Design review of the part built by this model. Coordinates are the model's own, in mm. Round coordinates to 2 decimals unless told otherwise and drop trailing zeros. Loops run counter-clockwise (first coordinate to the right, second up) from the corner with the lowest first, then second, coordinate; pieces in that order, holes last. Notation, with made-up numbers: (-21, 75) - (35, 75) arc R19 ccw to (35, 80) - close; hole circle Ø10 at (-25.75, 63.25). An arc over 180 degrees is marked (long way). Return JSON: item names as keys, results as strings. Group by question number.
(1) Wall thickness on L1, parallel to Y at x = 48, z = 4.7; L2, parallel to Y at x = -96, z = 2.35; L3, parallel to X at y = 65.5, z = 1.4: over which ranges is each line inside the solid? List them lowest first. Write a range as [from, to].
(2) We need section C-C, the plane x = 0. Write out the cut boundary in (y, z), and give its area (3 significant figures).
(3) We need section A-A, the plane x = -96. Write out the cut boundary in (y, z).
(4) Clearance check with flat-ended pins moving along their axes: pin 1 (1.8 mm diameter, centred on x = 29.5, z = 4.5, fed in from -Y); pin 2 (1 mm diameter, centred on y = -33.5, z = 4.5, fed in from -X); pin 3 (1.8 mm diameter, centred on y = -31.5, z = 4, fed in from +X). State where each tip first meets the part, or that it passes through.
(5) We need section B-B, the plane z = 1.75. Write out the cut boundary in (x, y).
(6) We need section D-D, the plane y = 63. Write out the cut boundary in (x, z), and give its area (3 significant figures).
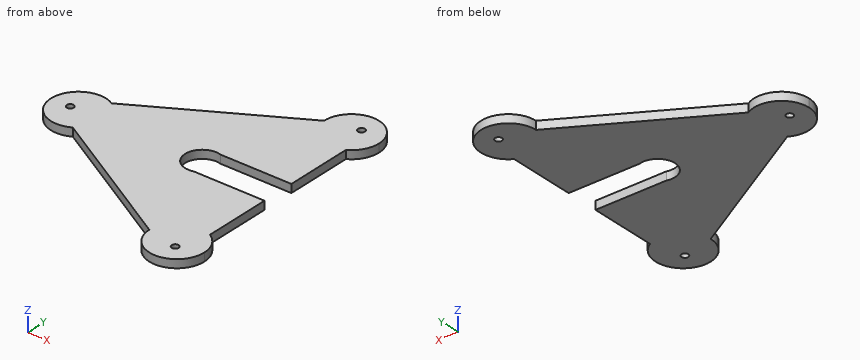
from build123d import *

# Parameters (mm, degrees)
F1_DEPTH        = 6
F2_R            = 12.5
F3_DEPTH        = 6
F4_R            = 2.5
F5_DEPTH        = 6
F5_COPIES_COUNT = 3
F6_W            = 60
F6_H            = 24
F7_DEPTH        = 6


# Not quite as in the source:
# - a pattern or mirror of a feature is missing from the dataset's text; its kind, count and spacing are read off the source's solid


with BuildPart() as f1:
    # F0 (on Top) → F1 (new body)
    with BuildSketch(Plane.XY):
        with BuildLine():
            ThreePointArc((-80, 17.3205080757), (-100, 17.3205080757), (-110, 0))
            Line((-110, 0), (-80, 17.3205080757))
        make_face()
        with BuildLine():
            Line((-80, 17.3205080757), (-110, 0))
            Line((-110, 0), (-80, -17.3205080757))
            ThreePointArc((-80, -17.3205080757), (-72.6794919243, -10), (-70, 0))
            ThreePointArc((-70, 0), (-72.6794919243, 10), (-80, 17.3205080757))
        make_face()
        with BuildLine():
            Line((-80, -17.3205080757), (-110, 0))
            ThreePointArc((-110, 0), (-100, -17.3205080757), (-80, -17.3205080757))
        make_face()
        with BuildLine():
            Line((25, 77.9422863406), (-80, 17.3205080757))
            ThreePointArc((-80, 17.3205080757), (-72.6794919243, 10), (-70, 0))
            ThreePointArc((-70, 0), (-72.6794919243, -10), (-80, -17.3205080757))
            Line((-80, -17.3205080757), (25, -77.9422863406))
            ThreePointArc((25, -77.9422863406), (35, -60.6217782649), (55, -60.6217782649))
            Line((55, -60.6217782649), (55, 60.6217782649))
            ThreePointArc((55, 60.6217782649), (35, 60.6217782649), (25, 77.9422863406))
        make_face()
        with BuildLine():
            ThreePointArc((55, 95.2627944163), (35, 95.2627944163), (25, 77.9422863406))
            Line((25, 77.9422863406), (55, 95.2627944163))
        make_face()
        with BuildLine():
            Line((55, 95.2627944163), (25, 77.9422863406))
            ThreePointArc((25, 77.9422863406), (35, 60.6217782649), (55, 60.6217782649))
            Line((55, 60.6217782649), (55, 95.2627944163))
        make_face()
        with BuildLine():
            ThreePointArc((55, -60.6217782649), (35, -60.6217782649), (25, -77.9422863406))
            Line((25, -77.9422863406), (55, -95.2627944163))
            Line((55, -95.2627944163), (55, -60.6217782649))
        make_face()
        with BuildLine():
            Line((55, -95.2627944163), (25, -77.9422863406))
            ThreePointArc((25, -77.9422863406), (35, -95.2627944163), (55, -95.2627944163))
        make_face()
        with BuildLine():
            ThreePointArc((65, 77.9422863406), (62.3205080757, 87.9422863406), (55, 95.2627944163))
            Line((55, 95.2627944163), (55, 60.6217782649))
            ThreePointArc((55, 60.6217782649), (62.3205080757, 67.9422863406), (65, 77.9422863406))
        make_face()
        with BuildLine():
            Line((55, -60.6217782649), (55, -95.2627944163))
            ThreePointArc((55, -95.2627944163), (62.3205080757, -87.9422863406), (65, -77.9422863406))
            ThreePointArc((65, -77.9422863406), (62.3205080757, -67.9422863406), (55, -60.6217782649))
        make_face()
    extrude(amount=F1_DEPTH)

    # F2 (on face) → F3 (cut, through all)
    with BuildSketch(Plane.XY.offset(6)):
        Circle(F2_R)
    extrude(amount=-F3_DEPTH, mode=Mode.SUBTRACT)

    # F4 (on face) → F5 (cut, through all)
    with BuildSketch(Plane.XY.offset(6)):
        with Locations((-96, 0)):
            Circle(F4_R)
    f5 = extrude(amount=-F5_DEPTH, mode=Mode.SUBTRACT)

    # F5_copies: F5 ×3 about axis
    f5_copies_axis = Axis((0, 0, 0), (0, 0, 1))
    for i in range(1, F5_COPIES_COUNT):
        add(f5.rotate(f5_copies_axis, i * 360 / F5_COPIES_COUNT), mode=Mode.SUBTRACT)

    # F6 (on face) → F7 (cut, through all)
    with BuildSketch(Plane.XY.offset(6)):
        with Locations((33.5, 0)):
            Rectangle(F6_W, F6_H)
    extrude(amount=-F7_DEPTH, mode=Mode.SUBTRACT)


solid = f1.part
Solutions:
{
 "1": {"L1": "[-97.72, -85.64], [-80.64, -12], [12, 80.64], [85.64, 97.72]", "L2": "[-19.08, -2.5], [2.5, 19.08]", "L3": "[3.45, 60.66]"},
 "2": {"outline": "(-63.51, 0) - (-12.5, 0) - (-12.5, 6) - (-63.51, 6) - close; (12.5, 0) - (63.51, 0) - (63.51, 6) - (12.5, 6) - close", "area": "612 mm^2"},
 "3": {"outline": "(-19.08, 0) - (-2.5, 0) - (-2.5, 6) - (-19.08, 6) - close; (2.5, 0) - (19.08, 0) - (19.08, 6) - (2.5, 6) - close"},
 "4": {"pin 1": "y = -91.61", "pin 2": "x = -52.84", "pin 3": "x = 55"},
 "5": {"outline": "(-80, -17.32) - (25, -77.94) arc R20 ccw (long way) to (55, -60.62) - (55, -12) - (3.5, -12) arc R12.5 cw (long way) to (3.5, 12) - (55, 12) - (55, 60.62) arc R20 ccw (long way) to (25, 77.94) - (-80, 17.32) arc R20 ccw (long way) to start; hole circle Ø5 at (-96, 0); hole circle Ø5 at (48, -83.14); hole circle Ø5 at (48, 83.14)"},
 "6": {"outline": "(-0.88, 0) - (58.29, 0) - (58.29, 6) - (-0.88, 6) - close", "area": "355 mm^2"}
}
